Design review of the part built by this model. Coordinates are the model's own, in mm. A direction names the side the tool comes from. Coordinates: 2 decimals unless noted, no trailing zeros. Loops run counter-clockwise (first coordinate to the right, second up) from the corner with the lowest first, then second, coordinate; pieces in that order, holes last.
Q1. Add section A-A on x = -25. Give the boundary of the cut face in (y, z).
Q2. For P1, Ø3, axis at x = -6, y = 11, coming from the -Z side, flat-tipped, find the tip position at first contact; note if it passes through.
Q3. Draft analysis for pull direction Z (two halves, no side actions). For faces 1 (the face through (-30, -9.238, 6)), 2 (the face through (0, 21, 0)), 3 (the face through (-15.233, -26, 6)), state which applies: released by +Z, released by -Z, zero draft, split by the parting line, or undercut.
Q4. Wall thickness on probe 1 along X at (y, z) = (9, 14); probe 2 along Y at (x, z) = (-20, 2); probe 3 along Z at (x, y) = (7.5, -11): over which ranges is each line inside the solid? List them lowest first.
Q5. Add section B-B on y = 22. Give the number of separate pieces and of enclosed holes in the cut face, and give its area (3 significant figures).
Q6. Machinability: for faces 4 (the face through (19.187, 0, 33)), 5 (the face through (11.767, 24, 5)), 6 (the face through (-14.656, -1, 32)), which of the approach directions +Z, -Z, +X, -X, +Y, -Y give a long, thin tool a straight path to every point of the face, cutting with its end or side? Answer none if there is none.
```python
from build123d import *

# Parameters (mm, degrees)
SKETCH2_W           = 57
SKETCH2_H           = 57
BOSS_EXTRUDE1_DEPTH = 35
SKETCH3_W           = 15
SKETCH3_H           = 2
CUT_EXTRUDE1_DEPTH  = 60
SKETCH4_W           = 42
SKETCH4_H           = 42
CUT_EXTRUDE2_DEPTH  = 28
CUT_EXTRUDE4_DEPTH  = 5
CUT_EXTRUDE5_DEPTH  = 10
CUT_EXTRUDE6_DEPTH  = 5
SKETCH13_W          = 7
SKETCH13_H          = 1.952566844
CUT_EXTRUDE8_DEPTH  = 12
SHELL3_START        = 21.262135922
SHELL3_OUTLINE_W    = 9
SHELL3_OUTLINE_H    = 3.952566844
SHELL3_DEPTH        = 5.5
SHELL3_START_2      = -28.237864078
SHELL3_2_DEPTH      = 18
SHELL3_START_3      = 8.762135922
SHELL3_3_DEPTH      = 12.5
SHELL3_4_DEPTH      = 5.5
SHELL3_START_4      = 16.266990291
SHELL3_5_OUTLINE_W  = 19
SHELL3_5_OUTLINE_H  = 29.761209032
SHELL3_5_DEPTH      = 5.5
SHELL3_START_5      = -14.656416284
SHELL3_6_OUTLINE_W  = 19
SHELL3_6_OUTLINE_H  = 5
SHELL3_6_DEPTH      = 17.843406575
SHELL3_START_6      = -33.233009709
SHELL3_7_DEPTH      = 5.5
SHELL3_START_7      = -27.733009709
SHELL3_8_OUTLINE_W  = 19
SHELL3_8_OUTLINE_H  = 1.76
SHELL3_8_DEPTH      = 44
SHELL3_START_8      = 20.186990291
SHELL3_9_OUTLINE_W  = 19
SHELL3_9_OUTLINE_H  = 3.238790968
SHELL3_9_DEPTH      = 1.58
SHELL3_10_OUTLINE_W = 19
SHELL3_10_OUTLINE_H = 3.24
SHELL3_10_DEPTH     = 1.576593425
SHELL3_START_9      = 3.186990291
SHELL3_11_OUTLINE_W = 19
SHELL3_11_OUTLINE_H = 0.001209032
SHELL3_11_DEPTH     = 13.08


with BuildPart() as part:
    # Sketch2 → Boss-Extrude1 (new body)
    with BuildSketch(Plane.XY):
        with Locations((-5.733009709, -0.737864078)):
            Rectangle(SKETCH2_W, SKETCH2_H)
    extrude(amount=BOSS_EXTRUDE1_DEPTH)

    # Sketch3 → Cut-Extrude1 (cut)
    with BuildSketch(Plane(origin=(0, 27.762135922, 0), x_dir=(1, 0, 0), z_dir=(0, 1, 0))):
        with Locations((-23.156416284, -32.76)):
            Rectangle(SKETCH3_W, SKETCH3_H)
        with Locations((11.686990291, -32.761209032)):
            Rectangle(SKETCH3_W, SKETCH3_H)
    extrude(amount=-CUT_EXTRUDE1_DEPTH, mode=Mode.SUBTRACT)

    # Sketch4 → Cut-Extrude2 (cut)
    with BuildSketch(Plane(origin=(0, 0, 0), x_dir=(-1, 0, 0), z_dir=(0, 0, -1))):
        with Locations((5.733009709, -0.737864078)):
            Rectangle(SKETCH4_W, SKETCH4_H)
    extrude(amount=-CUT_EXTRUDE2_DEPTH, mode=Mode.SUBTRACT)

    # Sketch5 → Cut-Extrude4 (cut)
    with BuildSketch(Plane(origin=(0, -21.737864078, 0), x_dir=(1, 0, 0), z_dir=(0, 1, 0))):
        with BuildLine():
            Line((2.766990291, -11), (2.766990291, 0))
            Line((2.766990291, 0), (-14.233009709, 0))
            Line((-14.233009709, 0), (-14.233009709, -11))
            ThreePointArc((-14.233009709, -11), (-5.733009709, -19.5), (2.766990291, -11))
        make_face()
    extrude(amount=-CUT_EXTRUDE4_DEPTH, mode=Mode.SUBTRACT)

    # Sketch7 → Cut-Extrude5 (cut)
    with BuildSketch(Plane(origin=(-26.733009709, 0, 0), x_dir=(0, 0, -1), z_dir=(1, 0, 0))):
        with BuildLine():
            Line((-11, -9.237864078), (0, -9.237864078))
            Line((0, -9.237864078), (0, 7.762135922))
            Line((0, 7.762135922), (-11, 7.762135922))
            ThreePointArc((-11, 7.762135922), (-19.5, -0.737864078), (-11, -9.237864078))
        make_face()
    extrude(amount=-CUT_EXTRUDE5_DEPTH, mode=Mode.SUBTRACT)

    # Sketch8 → Cut-Extrude6 (cut)
    with BuildSketch(Plane(origin=(0, -26.737864078, 0), x_dir=(1, 0, 0), z_dir=(0, 1, 0))):
        with BuildLine():
            Line((-14.233009709, 0), (2.766990291, 0))
            Line((2.766990291, 0), (2.766990291, -11))
            ThreePointArc((2.766990291, -11), (-5.733009709, -19.5), (-14.233009709, -11))
            Line((-14.233009709, -11), (-14.233009709, 0))
        make_face()
    extrude(amount=-CUT_EXTRUDE6_DEPTH, mode=Mode.SUBTRACT)

    # Sketch13 → Cut-Extrude8 (cut)
    with BuildSketch(Plane(origin=(0, 27.762135922, 0), x_dir=(1, 0, 0), z_dir=(0, 1, 0))):
        with Locations((8.266990291, -4.976283422)):
            Rectangle(SKETCH13_W, SKETCH13_H)
    extrude(amount=-CUT_EXTRUDE8_DEPTH, mode=Mode.SUBTRACT)

    # Shell3: read off the stored shape, not the designer's step
    # Shell3 outline → Shell3 (cut)
    with BuildSketch(Plane(origin=(0, 0, 0), x_dir=(1, 0, 0), z_dir=(0, 1, 0)).offset(SHELL3_START)):
        Polygon((-14.656416284, -30.76), (-14.656416284, -34), (3.186990291, -34), (3.186990291, -30.761209032), (20.186990291, -30.761209032), (20.186990291, -34), (21.766990291, -34), (21.766990291, -1), (-33.233009709, -1), (-33.233009709, -34), (-31.656416284, -34), (-31.656416284, -30.76), align=None)
        with Locations((8.266990291, -4.976283422)):
            Rectangle(SHELL3_OUTLINE_W, SHELL3_OUTLINE_H, mode=Mode.SUBTRACT)
    extrude(amount=SHELL3_DEPTH, mode=Mode.SUBTRACT)

    # Shell3 2 outline → Shell3 2 (cut)
    with BuildSketch(Plane(origin=(0, 0, 0), x_dir=(1, 0, 0), z_dir=(0, 1, 0)).offset(SHELL3_START_2)):
        Polygon((-14.656416284, -30.76), (-14.656416284, -34), (3.186990291, -34), (3.186990291, -30.761209032), (20.186990291, -30.761209032), (20.186990291, -34), (21.766990291, -34), (21.766990291, -1), (16.266990291, -1), (16.266990291, -29), (-27.733009709, -29), (-27.733009709, -1), (-33.233009709, -1), (-33.233009709, -34), (-31.656416284, -34), (-31.656416284, -30.76), align=None)
    extrude(amount=SHELL3_2_DEPTH, mode=Mode.SUBTRACT)

    # Shell3 3 outline → Shell3 3 (cut)
    with BuildSketch(Plane(origin=(0, 0, 0), x_dir=(1, 0, 0), z_dir=(0, 1, 0)).offset(SHELL3_START_3)):
        Polygon((-14.656416284, -30.76), (-14.656416284, -34), (3.186990291, -34), (3.186990291, -30.761209032), (20.186990291, -30.761209032), (20.186990291, -34), (21.766990291, -34), (21.766990291, -1), (16.266990291, -1), (16.266990291, -29), (-27.733009709, -29), (-27.733009709, -1), (-33.233009709, -1), (-33.233009709, -34), (-31.656416284, -34), (-31.656416284, -30.76), align=None)
    extrude(amount=SHELL3_3_DEPTH, mode=Mode.SUBTRACT)

    # Shell3 4 outline → Shell3 4 (cut)
    with BuildSketch(Plane(origin=(0, 0, 0), x_dir=(1, 0, 0), z_dir=(0, 1, 0)).offset(SHELL3_START_2)):
        with BuildLine():
            Line((-15.233009709, -1), (-27.733009709, -1))
            Line((-27.733009709, -1), (-27.733009709, -29))
            Line((-27.733009709, -29), (16.266990291, -29))
            Line((16.266990291, -29), (16.266990291, -1))
            Line((16.266990291, -1), (3.766990291, -1))
            Line((3.766990291, -1), (3.766990291, -11))
            ThreePointArc((3.766990291, -11), (-5.733009709, -20.5), (-15.233009709, -11))
            Line((-15.233009709, -11), (-15.233009709, -1))
        make_face()
    extrude(amount=SHELL3_4_DEPTH, mode=Mode.SUBTRACT)

    # Shell3 5 outline → Shell3 5 (cut)
    with BuildSketch(Plane.YZ.offset(SHELL3_START_4)):
        with Locations((-0.737864078, 15.880604516)):
            Rectangle(SHELL3_5_OUTLINE_W, SHELL3_5_OUTLINE_H)
    extrude(amount=SHELL3_5_DEPTH, mode=Mode.SUBTRACT)

    # Shell3 6 outline → Shell3 6 (cut)
    with BuildSketch(Plane.YZ.offset(SHELL3_START_5)):
        with Locations((-0.737864078, 31.5)):
            Rectangle(SHELL3_6_OUTLINE_W, SHELL3_6_OUTLINE_H)
    extrude(amount=SHELL3_6_DEPTH, mode=Mode.SUBTRACT)

    # Shell3 7 outline → Shell3 7 (cut)
    with BuildSketch(Plane.YZ.offset(SHELL3_START_6)):
        with BuildLine():
            Line((8.762135922, 30.76), (-10.237864078, 30.76))
            Line((-10.237864078, 30.76), (-10.237864078, 11))
            ThreePointArc((-10.237864078, 11), (-0.737864078, 20.5), (8.762135922, 11))
            Line((8.762135922, 11), (8.762135922, 30.76))
        make_face()
    extrude(amount=SHELL3_7_DEPTH, mode=Mode.SUBTRACT)

    # Shell3 8 outline → Shell3 8 (cut)
    with BuildSketch(Plane.YZ.offset(SHELL3_START_7)):
        with Locations((-0.737864078, 29.88)):
            Rectangle(SHELL3_8_OUTLINE_W, SHELL3_8_OUTLINE_H)
    extrude(amount=SHELL3_8_DEPTH, mode=Mode.SUBTRACT)

    # Shell3 9 outline → Shell3 9 (cut)
    with BuildSketch(Plane.YZ.offset(SHELL3_START_8)):
        with Locations((-0.737864078, 32.380604516)):
            Rectangle(SHELL3_9_OUTLINE_W, SHELL3_9_OUTLINE_H)
    extrude(amount=SHELL3_9_DEPTH, mode=Mode.SUBTRACT)

    # Shell3 10 outline → Shell3 10 (cut)
    with BuildSketch(Plane.YZ.offset(SHELL3_START_6)):
        with Locations((-0.737864078, 32.38)):
            Rectangle(SHELL3_10_OUTLINE_W, SHELL3_10_OUTLINE_H)
    extrude(amount=SHELL3_10_DEPTH, mode=Mode.SUBTRACT)

    # Shell3 11 outline → Shell3 11 (cut)
    with BuildSketch(Plane.YZ.offset(SHELL3_START_9)):
        with Locations((-0.737864078, 30.760604516)):
            Rectangle(SHELL3_11_OUTLINE_W, SHELL3_11_OUTLINE_H)
    extrude(amount=SHELL3_11_DEPTH, mode=Mode.SUBTRACT)


solid = part.part
```
Entries:
1. outline: (-29.24, 0) - (-21.74, 0) - (-21.74, 28) - (20.26, 28) - (20.26, 0) - (27.76, 0) - (27.76, 31.76) - (-29.24, 31.76) - close; (-29.24, 33.76) - (27.76, 33.76) - (27.76, 35) - (-29.24, 35) - close; hole (-28.24, 1) - (-22.74, 1) - (-22.74, 29) - (21.26, 29) - (21.26, 1) - (26.76, 1) - (26.76, 30.76) - (-28.24, 30.76) - close
2. P1: stops at z = 28
3. face 1: zero draft
3. face 2: released by -Z
3. face 3: undercut
4. probe 1: x = -34.23 to -33.23, -27.73 to -26.73, 15.27 to 16.27, 21.77 to 22.77
4. probe 2: y = -29.24 to -28.24, -22.74 to -21.74, 20.26 to 21.26, 26.76 to 27.76
4. probe 3: z = 28 to 29, 30.76 to 31.76, 33.76 to 35
5. separate pieces: 2
5. enclosed holes: 4
5. area: 252 mm2
6. face 4: +Y, -Y
6. face 5: +Y
6. face 6: none
